Work out the finished part from the listing and answer in its coordinate system (mm). A direction names the side the tool comes from. Coordinates: 2 decimals unless noted, no trailing zeros. Order: outer loops, then holes, each group sorted by start corner. A loop starts at its lowest first (then second) coordinate and runs counter-clockwise, first axis right, second up.
```python
from build123d import *

# Parameters (mm, degrees)
F1_DEPTH = 50
F3_W     = 72.638307
F3_H     = 53.745832
F4_DEPTH = 5
F5_W     = 72.638307
F5_H     = 53.745832
F6_DEPTH = 5


with BuildPart() as f1:
    # F0 (on Top) → F1 (new body)
    with BuildSketch(Plane.XY):
        Polygon((-39.250743, -16.938083), (-34.039024, -16.938083), (-34.039024, 30.293103), (27.524386, 30.293103), (27.524386, -16.938083), (33.387564, -16.938083), (33.387564, 36.807749), (-39.250743, 36.807749), align=None)
    extrude(amount=F1_DEPTH)

    # F3 (on offset) → F4 (join)
    with BuildSketch(Plane.XY.offset(50)):
        with Locations((-2.93159, 9.934833)):
            Rectangle(F3_W, F3_H)
    extrude(amount=-F4_DEPTH)

    # F5 (on Top) → F6 (join)
    with BuildSketch(Plane.XY):
        with Locations((-2.93159, 9.934833)):
            Rectangle(F5_W, F5_H)
    extrude(amount=F6_DEPTH)


solid = f1.part
```
1. The part is cut by section B-B (x = -13). Determine the outline of the cut face in (y, z), plus the area to 3 significant figures.
2. Consider probe 1 along X at (y, z) = (12, 34.5); probe 2 along Z at (x, y) = (-28.5, -14); probe 3 along Y at (x, z) = (3, 16). Determine where each line is inside the solid, lowest interval first.
3. The part is cut by section C-C (z = 26.5). Determine the outline of the cut face in (x, y).
4. The part is cut by section A-A (y = 19). Determine the outline of the cut face in (x, z), plus the area to 3 significant figures.
5. For faces 4 (the flat face through (-4, 7, 5)), 5 (the flat face through (-39.251, 10, 25)), determine the directions among +Z, -Z, +X, -X, +Y, -Y from which every point of the face is accessible in a straight line to the end or side of a thin tool.
6. The mould has two halves that part along X. Classify faces 1 (the flat face through (-39.251, 10, 48)), 2 (the flat face through (33.388, 10, 25)), 3 (the flat face through (-34.039, 6, 25)): released by +X, released by -X, zero draft, split by the parting line, or undercut.
7. A flat-ended cylindrical pin translates along its axis: pin 1 (5 mm diameter, centred on x = 0, z = 39, fed in from -Y). Find the tip coordinate at first contact, or state that the pin passes through.
Worked out:
1. outline: (-16.94, 0) - (36.81, 0) - (36.81, 50) - (-16.94, 50) - (-16.94, 45) - (30.29, 45) - (30.29, 5) - (-16.94, 5) - close
1. area: 798 mm2
2. probe 1: x = -39.25 to -34.04, 27.52 to 33.39
2. probe 2: z = 0 to 5, 45 to 50
2. probe 3: y = 30.29 to 36.81
3. outline: (-39.25, -16.94) - (-34.04, -16.94) - (-34.04, 30.29) - (27.52, 30.29) - (27.52, -16.94) - (33.39, -16.94) - (33.39, 36.81) - (-39.25, 36.81) - close
4. outline: (-39.25, 0) - (33.39, 0) - (33.39, 50) - (-39.25, 50) - close; hole (-34.04, 5) - (27.52, 5) - (27.52, 45) - (-34.04, 45) - close
4. area: 1,170 mm2
5. face 4: -Y
5. face 5: +Z, -Z, -X, +Y, -Y
6. face 1: released by -X
6. face 2: released by +X
6. face 3: undercut
7. pin 1: stops at y = 30.29
